Source: CAD feature listing. Evaluate the final solid. Frame: model axes, mm. A direction names the side the tool comes from. Round coordinates to 2 decimals unless told otherwise and drop trailing zeros. Loops run counter-clockwise (first coordinate to the right, second up) from the corner with the lowest first, then second, coordinate; pieces in that order, holes last. Notation, with made-up numbers: (9, 61.25) -> (25, 61.25) arc R32 ccw to (25, 90.25) -> close; hole circle Ø2 at (-33.5, -13.5). An arc over 180 degrees is marked (long way). Put each result on its own line as item: value. Start each with the question number.
1. Cut plane B-B (y = -2.25). Return the cut outline in (x, z).
2. Cut plane A-A (x = -1). Return the cut outline in (y, z).
3. Draft query along Z for faces 6 (the flat face through (-18.938, 10, 2)), 7 (the flat face through (-5, 3, 0)), 8 (the cylindrical face through (-14.82, 12.94, 2.46)). Return one class per face: pulls with the +Z half, pulls with the -Z half, needs draft (parallel to the pull), parting line crosses it, or undercut.
4. Cut plane C-C (z = 2.6). Return the cut outline in (x, y).
5. Material intervals for L1, parallel to X at y = 5.25, z = 2.55; L2, parallel to X at y = 4.75, z = 4.45; L3, parallel to Y at x = -19.5, z = 1.55, sorted ascending.
6. Contact query for flat-ended pins moving along their axis: pin 1 (2 mm diameter, centred on y = -5.38, z = 2.5, fed in from +X); pin 2 (3 mm diameter, centred on x = -8, y = 8.5, fed in from +Z). Output: stop coordinate, or through.
7. Set-up query: faces 1 (the flat face through (-21, 12.624, 2)), 2 (the flat face through (-9, 8, 1)), 3 (the cylindrical face through (-21.47, 10, 3.69)), 4 (the flat face through (-3, -8.376, 2)), 5 (the cylindrical face through (-4.437, -0.019, 2.465)). Return all of +Z, -Z, +X, -X, +Y, -Y with unobstructed straight access to the full face (end or side cutting, diameter ignored); none if empty.
```python
from build123d import *

# Parameters (mm, degrees)
SKETCH1_R           = 0.8
SKETCH1_R_2         = 5.1
BOSS_EXTRUDE1_DEPTH = 5
SKETCH2_R           = 1.25
CUT_EXTRUDE1_DEPTH  = 5
SKETCH21_R          = 5.1
BOSS_EXTRUDE2_DEPTH = 1


with BuildPart() as part:
    # Sketch1 → Boss-Extrude1 (new body)
    with BuildSketch(Plane(origin=(0, 0, 0), x_dir=(0, 1, 0), z_dir=(0, 0, 1))):
        with BuildLine():
            ThreePointArc((7.923715338, -23.061842121), (11.348253353, -21.704991773), (12.914157128, -18.370857874))
            Line((12.914157128, -18.370857874), (14.611258571, 9.036437401))
            ThreePointArc((14.611258571, 9.036437401), (14.470096631, 10.842810788), (13.835805455, 12.540039768))
            ThreePointArc((13.835805455, 12.540039768), (12.931450551, 14.850335933), (12.623684243, 17.312165753))
            Line((12.623684243, 17.312165753), (12.623684243, 23.938157879))
            Line((12.623684243, 23.938157879), (-8.376315757, 23.938157879))
            Line((-8.376315757, 23.938157879), (-8.376315757, -18.061842121))
            ThreePointArc((-8.376315757, -18.061842121), (-6.911849663, -21.597376027), (-3.376315757, -23.061842121))
            Line((-3.376315757, -23.061842121), (7.923715338, -23.061842121))
        make_face()
        with BuildLine():
            Line((-6.37591859, -2.133696229), (-6.376315757, -2.061842121))
            ThreePointArc((-6.376315757, -2.061842121), (0.123684243, 4.438157879), (6.623684243, -2.061842121))
            Line((6.623684243, -2.061842121), (6.623684243, -15.061842121))
            ThreePointArc((6.623684243, -15.061842121), (0.625179068, -21.542467318), (-6.298932046, -16.061842121))
            ThreePointArc((-6.298932046, -16.061842121), (-6.376216465, -15.097769724), (-6.309594086, -14.132901895))
            Line((-6.309594086, -14.132901895), (-6.37591859, -2.133696229))
        make_face(mode=Mode.SUBTRACT)
        with Locations(Location((9.123684243, -16.061842121, 0), (0, 0, 270))):
            Circle(SKETCH1_R, mode=Mode.SUBTRACT)
        with Locations(Location((9.623684243, -10.061842121, 0), (0, 0, 270))):
            Circle(SKETCH1_R, mode=Mode.SUBTRACT)
        with Locations(Location((9.123684243, -4.061842121, 0), (0, 0, 270))):
            Circle(SKETCH1_R, mode=Mode.SUBTRACT)
        with Locations(Location((8.123684243, 9.438157879, 0), (0, 0, 270))):
            Circle(SKETCH1_R_2, mode=Mode.SUBTRACT)
        with Locations(Location((4.623684243, 21.438157879, 0), (0, 0, 270))):
            Circle(SKETCH1_R, mode=Mode.SUBTRACT)
    extrude(amount=BOSS_EXTRUDE1_DEPTH)

    # Sketch2 → Cut-Extrude1 (cut)
    with BuildSketch(Plane(origin=(-23.938157879, 0, 0), x_dir=(0, -1, 0), z_dir=(-1, 0, 0))):
        with Locations(Location((-9.623684243, 2.5, 0), (0, 0, 90))):
            Circle(SKETCH2_R)
        with Locations(Location((5.376315757, 2.5, 0), (0, 0, 90))):
            Circle(SKETCH2_R)
    extrude(amount=-CUT_EXTRUDE1_DEPTH, mode=Mode.SUBTRACT)

    # Sketch21 → Boss-Extrude2 (add)
    with BuildSketch(Plane(origin=(0, 0, 0), x_dir=(1, 0, 0), z_dir=(0, 0, -1))):
        with Locations(Location((-9.438157879, -8.123684243, 0), (0, 0, 180))):
            Circle(SKETCH21_R)
    extrude(amount=-BOSS_EXTRUDE2_DEPTH)


solid = part.part
```
Solution:
1. outline: (-23.94, 0) -> (-3.99, 0) -> (-3.99, 5) -> (-23.94, 5) -> close; (21.11, 0) -> (23.06, 0) -> (23.06, 5) -> (21.11, 5) -> close
2. outline: (-8.38, 0) -> (-5.61, 0) -> (-5.61, 5) -> (-8.38, 5) -> close; (5.86, 0) -> (14.11, 0) -> (14.11, 5) -> (5.86, 5) -> close
3. face 6: undercut
3. face 7: pulls with the -Z half
3. face 8: needs draft
4. outline: (-23.94, -8.38) -> (18.06, -8.38) arc R5 ccw to (23.06, -3.38) -> (23.06, 7.92) arc R5 ccw to (18.37, 12.91) -> (-9.04, 14.61) arc R6.5 ccw to (-12.54, 13.84) arc R10 cw to (-17.31, 12.62) -> (-23.94, 12.62) -> (-23.94, 10.87) -> (-18.94, 10.87) -> (-18.94, 8.38) -> (-23.94, 8.38) -> (-23.94, -4.13) -> (-18.94, -4.13) -> (-18.94, -6.62) -> (-23.94, -6.62) -> close; hole circle Ø1.6 at (-21.44, 4.62); hole circle Ø10.2 at (-9.44, 8.12); hole (2.06, -6.38) -> (14.13, -6.31) arc R6.5 ccw (long way) to (15.06, 6.62) -> (2.06, 6.62) arc R6.5 ccw to start; hole circle Ø1.6 at (4.06, 9.12); hole circle Ø1.6 at (10.06, 9.62); hole circle Ø1.6 at (16.06, 9.12)
5. L1: x = -23.94 to -21.94, -20.94 to -13.65, -5.22 to -1.93, 19.06 to 23.06
5. L2: x = -23.94 to -22.23, -20.65 to -13.26, -5.61 to -2.5, 19.63 to 23.06
5. L3: y = -8.38 to -6.19, -4.56 to 8.81, 10.44 to 12.62
6. pin 1: stops at x = 22.96
6. pin 2: stops at z = 1
7. face 1: +Z, -Z, -X, +Y
7. face 2: +Z
7. face 3: -X
7. face 4: +Z, -Z, +X, -X, -Y
7. face 5: +Z, -Z
